Build history of the part. All positions in model axes, mm. A direction names the side the tool comes from. Give positions to 0.01 mm unless a question says otherwise; leave off trailing zeros. Order: outer loops, then holes, each group sorted by start corner. A loop starts at its lowest first (then second) coordinate and runs counter-clockwise, first axis right, second up. Notation, with made-up numbers: (-19, 57) - (-12, 57) arc R19 cw to (-12, 64) - close; hole circle Ø7 at (72.25, 85.5). An arc over 180 degrees is marked (long way). Answer in a Markdown table with one row per item.
```python
from build123d import *

# Parameters (mm, degrees)
SKETCH_1_W                 = 42.5
SKETCH_1_H                 = 35.5
EXTRUDE_1_DEPTH            = 40
SKETCH_2_W                 = 42.5
SKETCH_2_H                 = 35.5
SKETCH_2_W_2               = 30
SKETCH_2_H_2               = 21
CUT_EXTRUDE_1_DEPTH        = 7.3
SKETCH_3_W                 = 13
SKETCH_3_H                 = 26.5
EXTRUDE_2_DEPTH            = 2
EXTRUDE_3_DEPTH            = 0.8
EXTRUDE_3_DEPTH_BACK       = 0.8
SKETCH_4_W                 = 4.3
SKETCH_4_H                 = 2.75
SKETCH_5_R                 = 1.25
CUT_EXTRUDE_2_DEPTH        = 2
SKETCH_6_W                 = 42.5
SKETCH_6_H                 = 35.5
CUT_EXTRUDE_3_DEPTH        = 11
SKETCH_7_W                 = 2.5
SKETCH_7_H                 = 2.5
CUT_EXTRUDE_4_DEPTH        = 8
SKETCH_8_W                 = 25.8
SKETCH_8_H                 = 4.25
SKETCH_8_H_2               = 6.75
CUT_EXTRUDE_5_DEPTH        = 11
CUT_EXTRUDE_6_DEPTH        = 3.5
SKETCH_10_W                = 2.1
SKETCH_10_H                = 4.65
SKETCH_10_W_2              = 2.28
SKETCH_10_W_3              = 0.939967479
CUT_EXTRUDE_7_DEPTH        = 3.5
SKETCH_11_R                = 0.35
EXTRUDE_4_DEPTH            = 3
PATTERN_LINEAR_1_COUNT     = 3
PATTERN_LINEAR_1_PITCH     = 5.08
PATTERN_LINEAR_1_COL_COUNT = 3
PATTERN_LINEAR_1_COL_PITCH = 5.08
CUT_EXTRUDE_START          = -3
SKETCH_12_R                = 0.35
CUT_EXTRUDE_8_DEPTH        = 3


with BuildPart() as part:
    # Эскиз1 → Вытянуть1 (new body)
    with BuildSketch(Plane.XY):
        Rectangle(SKETCH_1_W, SKETCH_1_H)
    extrude(amount=EXTRUDE_1_DEPTH)

    # Эскиз2 → Вырез-Вытянуть1 (cut)
    with BuildSketch(Plane.XY.offset(40)):
        Rectangle(SKETCH_2_W, SKETCH_2_H)
        Rectangle(SKETCH_2_W_2, SKETCH_2_H_2, mode=Mode.SUBTRACT)
    extrude(amount=-CUT_EXTRUDE_1_DEPTH, mode=Mode.SUBTRACT)

    # Эскиз3 → Вытянуть2 (add)
    with BuildSketch(Plane.XY.offset(32.7)):
        Rectangle(SKETCH_3_W, SKETCH_3_H)
    extrude(amount=EXTRUDE_2_DEPTH)

    # Эскиз4 → Вытянуть3 (add, two sides: drawn at the far end of the back side and taken through both)
    with BuildSketch(Plane(origin=(0, 0, 0), x_dir=(0, 0, -1), z_dir=(1, 0, 0)).offset(-EXTRUDE_3_DEPTH_BACK)):
        Polygon((-34.7, 10.5), (-39, 10.5), (-34.7, 13.153893026), align=None)
        with Locations((-36.85, -11.875)):
            Rectangle(SKETCH_4_W, SKETCH_4_H)
    extrude(amount=EXTRUDE_3_DEPTH + EXTRUDE_3_DEPTH_BACK)

    # Эскиз5 → Вырез-Вытянуть2 (cut)
    with BuildSketch(Plane.XY.offset(40)):
        with Locations((-6.5, 5.25)):
            Circle(SKETCH_5_R)
        with Locations((6.5, 5.25)):
            Circle(SKETCH_5_R)
        with Locations((6.5, -5.25)):
            Circle(SKETCH_5_R)
        with Locations((-6.5, -5.25)):
            Circle(SKETCH_5_R)
    extrude(amount=-CUT_EXTRUDE_2_DEPTH, mode=Mode.SUBTRACT)

    # Эскиз6 → Вырез-Вытянуть3 (cut)
    with BuildSketch(Plane(origin=(0, 0, 0), x_dir=(-1, 0, 0), z_dir=(0, 0, -1))):
        Rectangle(SKETCH_6_W, SKETCH_6_H)
        with BuildLine():
            Line((-17.75, 4.25), (-13.7, 4.25))
            Line((-13.7, 4.25), (-13.7, 16.5))
            Line((-13.7, 16.5), (13.7, 16.5))
            Line((13.7, 16.5), (13.7, 4.25))
            Line((13.7, 4.25), (17.75, 4.25))
            ThreePointArc((17.75, 4.25), (20.75, 1.25), (17.75, -1.75))
            Line((17.75, -1.75), (13.7, -1.75))
            Line((13.7, -1.75), (13.7, -16.5))
            Line((13.7, -16.5), (-13.7, -16.5))
            Line((-13.7, -16.5), (-13.7, -1.75))
            Line((-13.7, -1.75), (-17.75, -1.75))
            ThreePointArc((-17.75, -1.75), (-20.75, 1.25), (-17.75, 4.25))
        make_face(mode=Mode.SUBTRACT)
    extrude(amount=-CUT_EXTRUDE_3_DEPTH, mode=Mode.SUBTRACT)

    # Эскиз7 → Вырез-Вытянуть4 (cut)
    with BuildSketch(Plane(origin=(0, 0, 0), x_dir=(-1, 0, 0), z_dir=(0, 0, -1))):
        with Locations((17.25, 1.25)):
            Rectangle(SKETCH_7_W, SKETCH_7_H)
        with Locations((-17.25, 1.25)):
            Rectangle(SKETCH_7_W, SKETCH_7_H)
    extrude(amount=-CUT_EXTRUDE_4_DEPTH, mode=Mode.SUBTRACT)

    # Эскиз8 → Вырез-Вытянуть5 (cut)
    with BuildSketch(Plane(origin=(0, 0, 0), x_dir=(-1, 0, 0), z_dir=(0, 0, -1))):
        with Locations((0, 8.375)):
            Rectangle(SKETCH_8_W, SKETCH_8_H)
        with Locations((0, -7.125)):
            Rectangle(SKETCH_8_W, SKETCH_8_H_2)
    extrude(amount=-CUT_EXTRUDE_5_DEPTH, mode=Mode.SUBTRACT)

    # Эскиз9 → Вырез-Вытянуть6 (cut)
    with BuildSketch(Plane(origin=(0, 0, 0), x_dir=(-1, 0, 0), z_dir=(0, 0, -1))):
        Polygon((12.9, 16.5), (-12.9, 16.5), (-12.9, 10.5), (-12.1, 10.5), (-12.1, 15.15), (12.1, 15.15), (12.1, 10.5), (12.9, 10.5), align=None)
        Polygon((12.9, -10.5), (12.9, -16.5), (-12.9, -16.5), (-12.9, -10.5), (-12.1, -10.5), (-12.1, -15.15), (12.1, -15.15), (12.1, -10.5), align=None)
    extrude(amount=-CUT_EXTRUDE_6_DEPTH, mode=Mode.SUBTRACT)

    # Эскиз10 → Вырез-Вытянуть7 (cut)
    with BuildSketch(Plane(origin=(0, 0, 0), x_dir=(-1, 0, 0), z_dir=(0, 0, -1))):
        with Locations((-2.45, 12.825)):
            Rectangle(SKETCH_10_W, SKETCH_10_H)
        with Locations((2.54, 12.825)):
            Rectangle(SKETCH_10_W_2, SKETCH_10_H)
        with Locations((7.62, 12.825)):
            Rectangle(SKETCH_10_W_2, SKETCH_10_H)
        with Locations((12.02998374, 12.825)):
            Rectangle(SKETCH_10_W_3, SKETCH_10_H)
        with Locations((-12.02998374, 12.825)):
            Rectangle(SKETCH_10_W_3, SKETCH_10_H)
        with Locations((-7.62, 12.825)):
            Rectangle(SKETCH_10_W_2, SKETCH_10_H)
        with Locations((-7.62, -12.825)):
            Rectangle(SKETCH_10_W_2, SKETCH_10_H)
        with Locations((-12.02998374, -12.825)):
            Rectangle(SKETCH_10_W_3, SKETCH_10_H)
        with Locations((12.02998374, -12.825)):
            Rectangle(SKETCH_10_W_3, SKETCH_10_H)
        with Locations((7.62, -12.825)):
            Rectangle(SKETCH_10_W_2, SKETCH_10_H)
        with Locations((2.54, -12.825)):
            Rectangle(SKETCH_10_W_2, SKETCH_10_H)
        with Locations((-2.45, -12.825)):
            Rectangle(SKETCH_10_W, SKETCH_10_H)
    extrude(amount=-CUT_EXTRUDE_7_DEPTH, mode=Mode.SUBTRACT)

    # Эскиз11 → Вытянуть4 (add)
    with BuildSketch(Plane(origin=(0, 0, 0), x_dir=(-1, 0, 0), z_dir=(0, 0, -1))):
        with Locations((0, 12.7)):
            Circle(SKETCH_11_R)
        with Locations(Location((0, -12.7, 0), (0, 0, 180))):
            Circle(SKETCH_11_R)
    extrude_4 = extrude(amount=EXTRUDE_4_DEPTH)

    # Линейный массив1: Вытянуть4 ×3
    with Locations(*[(i * PATTERN_LINEAR_1_PITCH, 0, 0) for i in range(1, PATTERN_LINEAR_1_COUNT)]):
        add(extrude_4)

    # Линейный массив1 col: Вытянуть4 ×3
    with Locations(*[(-i * PATTERN_LINEAR_1_COL_PITCH, 0, 0) for i in range(1, PATTERN_LINEAR_1_COL_COUNT)]):
        add(extrude_4)

    # Эскиз12 → Вырез-Вытянуть8 (cut)
    with BuildSketch(Plane(origin=(0, 0, -3), x_dir=(-1, 0, 0), z_dir=(0, 0, -1)).offset(CUT_EXTRUDE_START)):
        with Locations((10.16, 12.7)):
            Circle(SKETCH_12_R)
        with Locations((10.16, -12.7)):
            Circle(SKETCH_12_R)
        with Locations((0, -12.7)):
            Circle(SKETCH_12_R)
        with Locations((-5.08, -12.7)):
            Circle(SKETCH_12_R)
    extrude(amount=CUT_EXTRUDE_8_DEPTH, mode=Mode.SUBTRACT)


solid = part.part
```
1. Probe line 1 (Y direction, x = -6.5, z = 39.1); line 2 (Y direction, x = 3.5, z = 5); line 3 (X direction, y = 8.5, z = 34). List the from-to ranges inside material, lowest first.
Check result:
| item | result |
|---|---|
| line 1 | y = -10.5 to -6.5, -4 to 4, 6.5 to 10.5 |
| line 2 | y = -16.5 to -10.5, -3.75 to 6.25, 10.5 to 16.5 |
| line 3 | x = -15 to 15 |
2. Two-plate mould, pull along X, no slides. Class faces 1 (the face through (-16, -1.75, 5)), 2 (the face through (6, 5, 38)), 3 (the face through (-0.8, -12, 37)), 4 (the face through (21.25, 0, 22)): +X half, -X half, draft (parallel to the pull), parting line (faces both ways), or undercut.
Check result:
| item | result |
|---|---|
| face 1 | draft |
| face 2 | undercut |
| face 3 | -X half |
| face 4 | +X half |
3. Drop flat-ended pins along their axis: P1, Ø12, axis at x = 9.5, y = 3, coming from the -Z side; P2, Ø2, axis at y = -8, z = 6.5, coming from the -X side; P3, Ø3, axis at x = 7, y = 13.5, coming from the +Z side. Give the stop position or say it passes through.
Check result:
| item | result |
|---|---|
| P1 | stops at z = 0 |
| P2 | stops at x = -13.7 |
| P3 | stops at z = 34.7 |
4. Cut at B-B on y = 5.25. Write the cut outline in (x, z), and give its area (3 significant figures).
Check result:
| item | result |
|---|---|
| outline | (-21.25, 11) - (-13.7, 11) - (-13.7, 0) - (13.7, 0) - (13.7, 11) - (21.25, 11) - (21.25, 32.7) - (15, 32.7) - (15, 40) - (7.75, 40) - (7.75, 38) - (5.25, 38) - (5.25, 40) - (-5.25, 40) - (-5.25, 38) - (-7.75, 38) - (-7.75, 40) - (-15, 40) - (-15, 32.7) - (-21.25, 32.7) - close |
| area | 1,430 mm² |
5. Which spindle directions (+Z, -Z, +X, -X, +Y, -Y) get a long thin tool onto all of the face, cutting with end or side? Do faces 5 (the face through (5.5, -6, 39)), 6 (the face through (-6.5, 12, 34)), 7 (the face through (-17, 1, 8)), 8 (the face through (3.5, 13, 2)). Say none if no direction does.
Check result:
| item | result |
|---|---|
| face 5 | +Z |
| face 6 | +Z, -X, +Y |
| face 7 | -Z |
| face 8 | -Z, +Y |
6. Cut at A-A on z = 2.5. Count the separate pieces of the cut face and the enclosed holes in it, and give its area (3 significant figures).
Check result:
| item | result |
|---|---|
| separate pieces | 11 |
| enclosed holes | 2 |
| area | 507 mm² |
